```python
from build123d import *

# Parameters (mm, degrees)
SKETCH1_W           = 82.2
SKETCH1_H           = 3.6
BOSS_EXTRUDE1_DEPTH = 82.2
SKETCH2_W           = 76.4
SKETCH2_H           = 76.4
CUT_EXTRUDE1_DEPTH  = 1.31
SKETCH4_R           = 1
CUT_EXTRUDE3_DEPTH  = 1.31
SKETCH3_W           = 46
SKETCH3_H           = 46
CUT_EXTRUDE2_DEPTH  = 92.930920261
SKETCH6_W           = 50.3
SKETCH6_H           = 50.3
CUT_EXTRUDE4_DEPTH  = 1.7
FILLET1_R           = 3
FILLET2_R           = 2


with BuildPart() as part:
    # Sketch1 → Boss-Extrude1 (new body)
    with BuildSketch(Plane(origin=(0, 0, 0), x_dir=(1, 0, 0), z_dir=(0, 1, 0))):
        with Locations((0, 1.8)):
            Rectangle(SKETCH1_W, SKETCH1_H)
    extrude(amount=BOSS_EXTRUDE1_DEPTH)

    # Sketch2 → Cut-Extrude1 (cut)
    with BuildSketch(Plane(origin=(0, 0, -3.6), x_dir=(-1, 0, 0), z_dir=(0, 0, -1))):
        with Locations((0, 41.1)):
            Rectangle(SKETCH2_W, SKETCH2_H)
    extrude(amount=-CUT_EXTRUDE1_DEPTH, mode=Mode.SUBTRACT)

    # Sketch4 → Cut-Extrude3 (cut)
    with BuildSketch(Plane(origin=(0, 0, -3.6), x_dir=(-1, 0, 0), z_dir=(0, 0, -1))):
        with Locations((38.2, 2.9)):
            Circle(SKETCH4_R)
        with Locations((38.2, 79.3)):
            Circle(SKETCH4_R)
        with Locations((-38.2, 2.9)):
            Circle(SKETCH4_R)
        with Locations((-38.2, 79.3)):
            Circle(SKETCH4_R)
    extrude(amount=-CUT_EXTRUDE3_DEPTH, mode=Mode.SUBTRACT)

    # Sketch3 → Cut-Extrude2 (cut, through all)
    with BuildSketch(Plane(origin=(0, 0, -2.29), x_dir=(-1, 0, 0), z_dir=(0, 0, -1))):
        with Locations((0, 41.1)):
            Rectangle(SKETCH3_W, SKETCH3_H)
    extrude(amount=-CUT_EXTRUDE2_DEPTH, mode=Mode.SUBTRACT)

    # Sketch6 → Cut-Extrude4 (cut)
    with BuildSketch(Plane.XY.offset(-2.29)):
        with Locations((0, 41.1)):
            Rectangle(SKETCH6_W, SKETCH6_H)
    extrude(amount=CUT_EXTRUDE4_DEPTH, mode=Mode.SUBTRACT)

    # Fillet1
    fillet1_edges = [part.edges().sort_by_distance(p)[0] for p in [
        (-41.1, 82.2, -1.8),
        (41.1, 82.2, -1.8),
        (-41.1, 0, -1.8),
        (41.1, 0, -1.8),
        (23, 18.1, -0.295),
        (23, 64.1, -0.295),
        (-23, 64.1, -0.295),
        (-23, 18.1, -0.295),
    ]]
    fillet(fillet1_edges, radius=FILLET1_R)

    # Fillet2
    fillet2_edges = [part.edges().sort_by_distance(p)[0] for p in [
        (-37.2, 79.3, -2.945),
        (-38.2, 78.3, -2.945),
        (38.2, 3.9, -2.945),
        (37.2, 2.9, -2.945),
        (38.2, 78.3, -2.945),
        (37.2, 79.3, -2.945),
        (-38.2, 3.9, -2.945),
        (-37.2, 2.9, -2.945),
    ]]
    fillet(fillet2_edges, radius=FILLET2_R)


solid = part.part
```
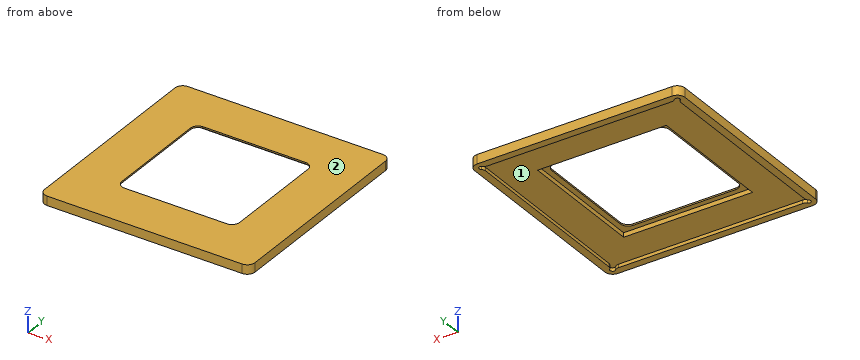
The listing builds one solid part. Answer for the finished solid, in the listing's coordinates (mm). Face numbers are marked on the shaded views. Give positions to 0.01 mm unless a question says otherwise; leave off trailing zeros. Order: outer loops, then holes, each group sorted by start corner. A loop starts at its lowest first (then second) coordinate and runs counter-clockwise, first axis right, second up. Notation, with made-up numbers: (-27.5, 9.5) -> (29.5, 9.5) arc R25 cw to (29.5, 40.5) -> close; hole circle Ø2 at (14.5, 33.5). An arc over 180 degrees is marked (long way). Write each question's results on one line, items separated by ' | '.
Q1. Straight lines are drawn through the part: probe 1 along X at (y, z) = (53.5, -3.3); probe 2 along Y at (x, z) = (27, -2.9); probe 3 along X at (y, z) = (66, -1.15). For each, find the intervals that lie inside material, in ascending order. Write a range as from..to.
Checked values:
probe 1: x = -41.1..-38.2, 38.2..41.1 | probe 2: y = 0..2.9, 79.3..82.2 | probe 3: x = -41.1..-25.15, 25.15..41.1
Q2. The part is cut by section C-C, the plane x = -33.5. Give the vertices of the cut face in (y, z).
Checked values:
outline: (0, -3.6) -> (2.9, -3.6) -> (2.9, -2.29) -> (79.3, -2.29) -> (79.3, -3.6) -> (82.2, -3.6) -> (82.2, 0) -> (0, 0) -> close
Q3. Determine the mould class of the marked faces 1 and 2 for opening direction X: pulls with the +X half, pulls with the -X half, needs draft (parallel to the pull), parting line crosses it, or undercut.
Checked values:
face 1: undercut | face 2: needs draft
Q4. The part is cut by section B-B, the plane y = 56. Give the vertices of the cut face in (x, z).
Checked values:
outline: (-41.1, -3.6) -> (-38.2, -3.6) -> (-38.2, -2.29) -> (-25.15, -2.29) -> (-25.15, -0.59) -> (-23, -0.59) -> (-23, 0) -> (-41.1, 0) -> close; (23, -0.59) -> (25.15, -0.59) -> (25.15, -2.29) -> (38.2, -2.29) -> (38.2, -3.6) -> (41.1, -3.6) -> (41.1, 0) -> (23, 0) -> close
Q5. Each of these flat-tipped pins is pushed along its axis until it touches: P1, Ø1, axis at x = -4, y = 66, coming from the -Z side; P2, Ø3, axis at x = -20, y = 46.5, coming from the +Z side. Where does it stop, or does it pass through?
Checked values:
P1: stops at z = -2.29 | P2: passes through
Q6. The part is cut by section A-A, the plane x = 2. Give the vertices of the cut face in (y, z).
Checked values:
outline: (0, -3.6) -> (2.9, -3.6) -> (2.9, -2.29) -> (15.95, -2.29) -> (15.95, -0.59) -> (18.1, -0.59) -> (18.1, 0) -> (0, 0) -> close; (64.1, -0.59) -> (66.25, -0.59) -> (66.25, -2.29) -> (79.3, -2.29) -> (79.3, -3.6) -> (82.2, -3.6) -> (82.2, 0) -> (64.1, 0) -> close
